Design review of the part built by this model. Coordinates are the model's own, in mm. A direction names the side the tool comes from. Give positions to 0.01 mm unless a question says otherwise; leave off trailing zeros. Write each loop counter-clockwise with the first axis right and the second up, starting at its lowest first coordinate (ties: lowest second). Pieces come first, ordered by that corner, then holes.
```python
from build123d import *

# Parameters (mm, degrees)
SKETCH_1_W          = 65
SKETCH_1_H          = 30.2
EXTRUDE_1_DEPTH     = 2
SKETCH_2_R          = 1.5
CUT_EXTRUDE_1_DEPTH = 3
FILLET_1_R          = 3.5
SKETCH_4_W          = 50.8
SKETCH_4_H          = 5.08
EXTRUDE_2_DEPTH     = 3


with BuildPart() as part:
    # 草圖1 → 填料-伸長1 (new body)
    with BuildSketch(Plane(origin=(0, 0, 0), x_dir=(1, 0, 0), z_dir=(0, 1, 0))):
        Rectangle(SKETCH_1_W, SKETCH_1_H)
    extrude(amount=EXTRUDE_1_DEPTH)

    # 草圖2 → 除料-伸長1 (cut, through all)
    with BuildSketch(Plane(origin=(0, 2, 0), x_dir=(1, 0, 0), z_dir=(0, 1, 0))):
        with Locations((-29, 11.6)):
            Circle(SKETCH_2_R)
        with Locations((-29, -11.4)):
            Circle(SKETCH_2_R)
        with Locations((29, -11.4)):
            Circle(SKETCH_2_R)
        with Locations((29, 11.6)):
            Circle(SKETCH_2_R)
    extrude(amount=-CUT_EXTRUDE_1_DEPTH, mode=Mode.SUBTRACT)

    # 圓角1
    fillet_1_edges = [part.edges().sort_by_distance(p)[0] for p in [
        (32.5, 1, 15.1),
        (-32.5, 1, 15.1),
        (-32.5, 1, -15.1),
        (32.5, 1, -15.1),
    ]]
    fillet(fillet_1_edges, radius=FILLET_1_R)

    # 草圖4 → 填料-伸長2 (add)
    with BuildSketch(Plane.XZ):
        with Locations((0, 11.06)):
            Rectangle(SKETCH_4_W, SKETCH_4_H)
    extrude(amount=EXTRUDE_2_DEPTH)


solid = part.part
```
(1) Consider section B-B, the plane y = -1.7. Give the boundary of the cut face in (x, z), then the cut area to 3 significant figures.
Resolved:
outline: (-25.4, 8.52) - (25.4, 8.52) - (25.4, 13.6) - (-25.4, 13.6) - close
area: 258 mm2
(2) Clearance check with flat-ended pins moving along their axes: P1, Ø1.8, axis at x = -29, z = -11.6, coming from the -Y side; P2, Ø1.5, axis at x = -20.5, z = -6.5, coming from the -Y side; P3, Ø0.9, axis at x = -7.5, y = -1, coming from the -Z side; P4, Ø2.5, axis at x = -5.5, y = -2, coming from the +Z side. State where each tip first meets the part, or that it passes through.
Resolved:
P1: passes through
P2: stops at y = 0
P3: stops at z = 8.52
P4: stops at z = 13.6
(3) Consider section A-A, the plane x = -5. Give the boundary of the cut face in (y, z).
Resolved:
outline: (-3, 8.52) - (0, 8.52) - (0, -15.1) - (2, -15.1) - (2, 15.1) - (0, 15.1) - (0, 13.6) - (-3, 13.6) - close
(4) Tool access review of faces 4 (the face through (25.4, -1, 11)), 5 (the face through (-25.4, -1, 11)), 6 (the face through (0, -1, 13.6)), 7 (the face through (0, -1, 8.52)): name each direction out of +Z, -Z, +X, -X, +Y, -Y from which nothing blocks a thin tool from reaching the whole face with its end or side.
Resolved:
face 4: +Z, -Z, +X, -Y
face 5: +Z, -Z, -X, -Y
face 6: +Z, +X, -X, -Y
face 7: -Z, +X, -X, -Y
(5) To check wall thickness, follow L1, parallel to Z at x = -29, y = 1.45; L2, parallel to X at y = 0.5, z = -11.6; L3, parallel to Y at x = 21.5, z = -1.5. State the ranges of each line that lie inside material, in increasing order.
Resolved:
L1: z = -15.1 to -13.1, -10.1 to 9.9, 12.9 to 15.1
L2: x = -32.5 to -30.5, -27.5 to 27.5, 30.5 to 32.5
L3: y = 0 to 2
(6) Mouldability with a two-part tool opening along X and no side actions: class faces 1 (the face through (-30.5, 1.01, 11.33)), 2 (the face through (0, 0, -4)), 3 (the face through (-31.5, 1.01, 14.05)) as pulls with the +X half, pulls with the -X half, needs draft (parallel to the pull), parting line crosses it, or undercut.
Resolved:
face 1: undercut
face 2: needs draft
face 3: pulls with the -X half
(7) Consider section C-C, the plane z = -2. Give the boundary of the cut face in (x, y), then the cut area to 3 significant figures.
Resolved:
outline: (-32.5, 0) - (32.5, 0) - (32.5, 2) - (-32.5, 2) - close
area: 130 mm2
